Verification items for this drawing (mm, ordinates from the low corner). A direction names the side the tool comes from. Give positions to 0.01 mm unless a question says otherwise; leave off trailing zeros. Order: outer loops, then holes, each group sorted by start corner. A loop starts at its lowest first (then second) coordinate and runs counter-clockwise, first axis right, second up.
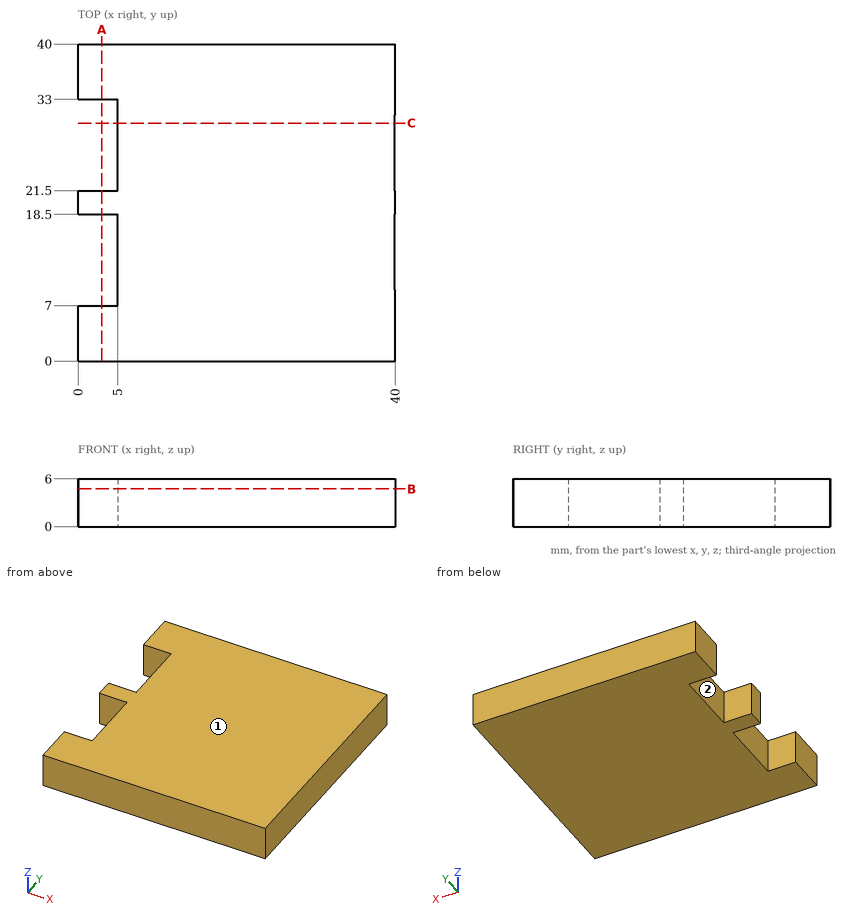
Q1. Gauge pin test, flat ends, axial feed: P1, Ø1.5, axis at x = 1.5, z = 4, coming from the -Y side; P2, Ø1.8, axis at y = 26.5, z = 3, coming from the -X side. Record the tip position at first contact, or that the pin passes through.
Q2. Cross-section at B-B, the plane z = 4.75. Record the boundary of the cut face in (x, y), and give its area (4 significant figures).
Q3. Access from +Z, -Z, +X, -X, +Y, -Y to the whole of each face (thin tool, end or side, straight path). Record for the marked faces 1 and 2.
Q4. Cross-section at A-A, the plane x = 3. Record the boundary of the cut face in (y, z), and give its area (3 significant figures).
Q5. Cross-section at C-C, the plane y = 30. Record the boundary of the cut face in (x, z).
Q6. Thickness scan on L1, parallel to Y at x = 2, z = 0.65; L2, parallel to X at y = 18, z = 3.45. Record the ranges inside material, lowest first.
Answers follow:
1. P1: stops at y = 0
1. P2: stops at x = 5
2. outline: (0, 0) - (40, 0) - (40, 40) - (0, 40) - (0, 33) - (5, 33) - (5, 21.5) - (0, 21.5) - (0, 18.5) - (5, 18.5) - (5, 7) - (0, 7) - close
2. area: 1,485 mm2
3. face 1: +Z, +X, -X, +Y, -Y
3. face 2: +Z, -Z, -X
4. outline: (0, 0) - (7, 0) - (7, 6) - (0, 6) - close; (18.5, 0) - (21.5, 0) - (21.5, 6) - (18.5, 6) - close; (33, 0) - (40, 0) - (40, 6) - (33, 6) - close
4. area: 102 mm2
5. outline: (5, 0) - (40, 0) - (40, 6) - (5, 6) - close
6. L1: y = 0 to 7, 18.5 to 21.5, 33 to 40
6. L2: x = 5 to 40
